from build123d import *

# Parameters (mm, degrees)
F0_R          = 10.7982965202
F1_DEPTH      = 86.614
F0_W          = 87.2836336493
F0_H          = 71.939252317
F2_DEPTH      = 35.306
F4_DEPTH      = 25.4
F4_DEPTH_BACK = 25.4


with BuildPart() as f1:
    # F0 (on Top) → F1 (new body)
    with BuildSketch(Plane.XY):
        with Locations((1.5942216851, 0)):
            Circle(F0_R)
    extrude(amount=F1_DEPTH)

    # F0 (on Top) → F2 (join)
    with BuildSketch(Plane.XY):
        Rectangle(F0_W, F0_H)
        with Locations((1.5942216851, 0)):
            Circle(F0_R, mode=Mode.SUBTRACT)
    extrude(amount=F2_DEPTH)

    # F3 (on Front) → F4 (cut, two sides)
    with BuildSketch(Plane.XZ) as f4_sk:
        Polygon((33.4245190024, 102.3935750127), (-31.5084643662, 97.7098867297), (33.4245190024, 50.4471883178), align=None)
    extrude(amount=-F4_DEPTH, mode=Mode.SUBTRACT)
    extrude(f4_sk.sketch, amount=F4_DEPTH_BACK, mode=Mode.SUBTRACT)


solid = f1.part
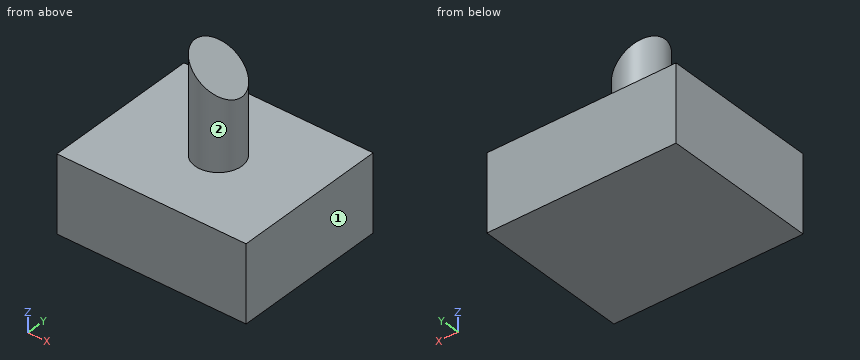
Source: CAD feature listing. Evaluate the final solid. Frame: model axes, mm. Face numbers are marked on the shaded views. A direction names the side the tool comes from. Give positions to 0.01 mm unless a question says otherwise; leave off trailing zeros. Write each loop counter-clockwise with the first axis right and the second up, starting at its lowest first coordinate (ties: lowest second). Pieces come first, ordered by that corner, then holes. Notation, with made-up numbers: (12, 81.5) -> (35, 81.5) arc R24 cw to (35, 96.5) -> close; hole circle Ø5 at (89, -39). An arc over 180 degrees is marked (long way). Return JSON: item names as keys, results as strings. Group by question number.
1. Section B-B, the plane x = -16. Output: boundary loops of the cut face in (y, z).
2. Section A-A, the plane y = 0. Output: boundary loops of the cut face in (x, z).
3. Section D-D, the plane y = 29.5. Output: boundary loops of the cut face in (x, z), then the cut area to 3 significant figures.
4. Section C-C, the plane z = 63. Output: boundary loops of the cut face in (x, y), then the cut area to 3 significant figures.
5. Material intervals for line 1 (Z direction, x = -19.5, y = -26.5); line 2 (Z direction, x = -4, y = 0); line 3 (X direction, y = 5.5, z = 46), sorted ascending. Write a range as from..to.
6. Pin query (flat end, axial travel): pin 1 Ø2 at (x, y) = (7.5, 14.5) entering from +Z; pin 2 Ø5 at (x, z) = (-2, 61) entering from -Y. Return the tip coordinate at first contact, or that it passes through.
7. Access query for the marked faces 1 and 2. Directions: +Z, -Z, +X, -X, +Y, -Y. A direction counts if a zero-diameter tool reaches every point of the face in a straight line with its end or side. Return the directions, or none.
Determined:
{
 "1": {"outline": "(-35.97, 0) -> (35.97, 0) -> (35.97, 35.31) -> (-35.97, 35.31) -> close"},
 "2": {"outline": "(-43.64, 0) -> (43.64, 0) -> (43.64, 35.31) -> (12.39, 35.31) -> (12.39, 65.76) -> (-9.2, 81.48) -> (-9.2, 35.31) -> (-43.64, 35.31) -> close"},
 "3": {"outline": "(-43.64, 0) -> (43.64, 0) -> (43.64, 35.31) -> (-43.64, 35.31) -> close", "area": "3,080 mm2"},
 "4": {"outline": "circle Ø21.6 at (1.59, 0)", "area": "366 mm2"},
 "5": {"line 1": "z = 0..35.31", "line 2": "z = 0..77.69", "line 3": "x = -7.7..10.89"},
 "6": {"pin 1": "stops at z = 35.31", "pin 2": "stops at y = -10.74"},
 "7": {"face 1": "+Z, -Z, +X, +Y, -Y", "face 2": "+Z"}
}
